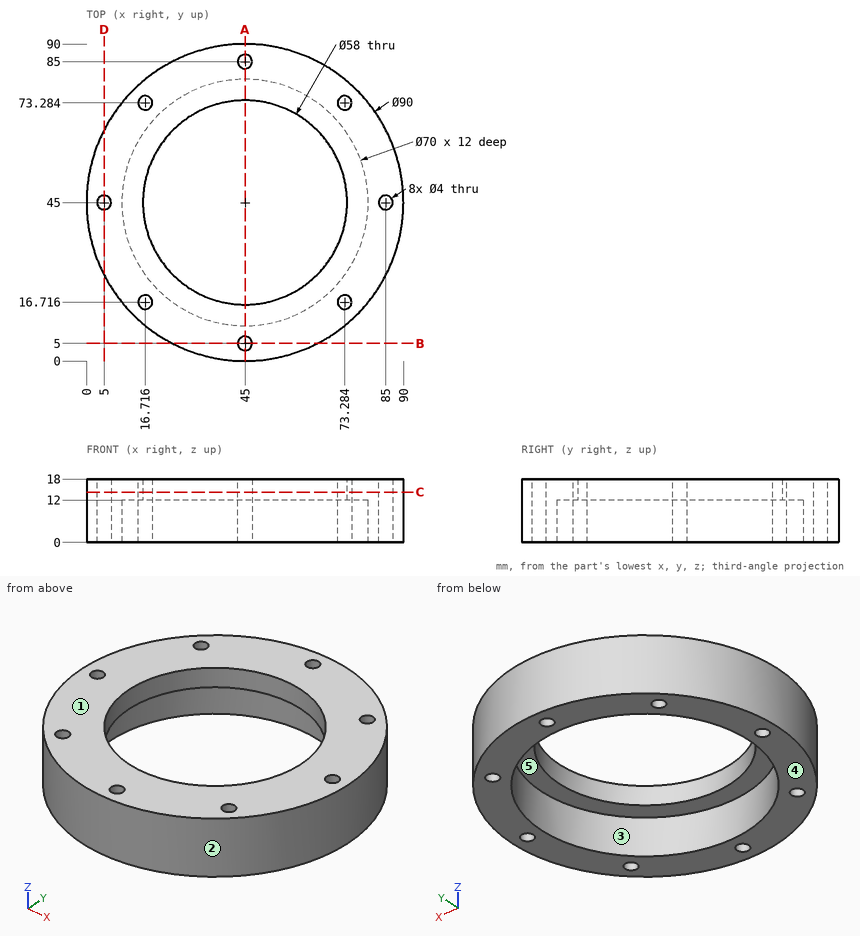
Could you check a few things on this drawing? It's one solid part, dimensions in mm from its lowest x, y, z. A direction names the side the tool comes from. Round coordinates to 2 decimals unless told otherwise and drop trailing zeros. Loops run counter-clockwise (first coordinate to the right, second up) from the corner with the lowest first, then second, coordinate; pieces in that order, holes last. Notation, with made-up numbers: (65.5, 54.5) -> (72.5, 54.5) arc R35 cw to (72.5, 90.5) -> close; hole circle Ø3 at (66.5, 6). An arc over 180 degrees is marked (long way). Write each question's results on one line, items separated by ' | '.
(1) We'd pull the mould along X, two halves only. Please class the marked faces 1, 2 and 3: released by +X, released by -X, zero draft, split by the parting line, or undercut.
Worked answers:
face 1: zero draft | face 2: split by the parting line | face 3: undercut
(2) If we section it at B-B, the plane y = 5: List the corners of the cut face in (x, z) for me (1 decimal).
Worked answers:
outline: (24.4, 0) -> (43, 0) -> (43, 18) -> (24.4, 18) -> close; (47, 0) -> (65.6, 0) -> (65.6, 18) -> (47, 18) -> close
(3) For P1, Ø8, axis at x = 71, z = 3.5, coming from the -Y side (1 decimal); P2, Ø8, axis at y = 50, z = 8.5, coming from the +X side; P3, Ø1.5, axis at x = 72, z = 14.5, coming from the +Y side, each with a flat end and sliding along its axis, tell me the tip position at first contact or that it passes through.
Worked answers:
P1: y = 5.7 | P2: x = 89.99 | P3: y = 81.55
(4) If I drill on L1, parallel to Y at x = 45, z = 13.9; L2, parallel to Y at x = 45, z = 8; L3, parallel to X at y = 46, z = 13, over which ranges is the centre line in solid material (lowest first)?
Worked answers:
L1: 0 to 3, 7 to 16, 74 to 83, 87 to 90 | L2: 0 to 3, 7 to 10, 80 to 83, 87 to 90 | L3: 0.01 to 3.27, 6.73 to 16.02, 73.98 to 83.27, 86.73 to 89.99
(5) If we section it at C-C, the plane z = 14.25: Give the number of separate pieces and of enclosed holes in the cut face, then the cut area to 3 significant figures.
Worked answers:
separate pieces: 1 | enclosed holes: 9 | area: 3,620 mm2
(6) For the marked faces 4 and 5, which set-ups out of +Z, -Z, +X, -X, +Y, -Y let a thin tool reach every point of the face, with its end or its side?
Worked answers:
face 4: -Z, +X, -X, +Y, -Y | face 5: -Z
(7) If we section it at A-A, the plane x = 45: List the corners of the cut face in (y, z) for me, then the cut area to 3 significant figures.
Worked answers:
outline: (0, 0) -> (3, 0) -> (3, 18) -> (0, 18) -> close; (7, 0) -> (10, 0) -> (10, 12) -> (16, 12) -> (16, 18) -> (7, 18) -> close; (74, 12) -> (80, 12) -> (80, 0) -> (83, 0) -> (83, 18) -> (74, 18) -> close; (87, 0) -> (90, 0) -> (90, 18) -> (87, 18) -> close | area: 288 mm2
